from build123d import *

# Parameters (mm, degrees)
F0_W         = 50
F0_H         = 16
F1_DEPTH     = 13
F2_W         = 6.1
F2_H         = 2
F2_H_2       = 16
F3_DEPTH     = 1
F5_D         = 2.5
F5_DEPTH     = 9.5
F5_TIP       = 0.7510757738
F6_SIZE      = 0.5
F8_DEPTH     = 50.001
F9_DEPTH     = 50.001
F10_T1_DEPTH = 22.4650386507
F10_T3_DEPTH = 22.5


# Not quite as in the source:
# - a fillet or chamfer that OpenCascade refuses, or shapes differently, is made with other operations: its cross-section is extruded or revolved along the edge and cut away or added


with BuildPart() as f1:
    # F0 (on Front) → F1 (new body)
    with BuildSketch(Plane.XZ):
        with Locations((25, 8)):
            Rectangle(F0_W, F0_H)
    extrude(amount=F1_DEPTH)

    # F2 (on face) → F3 (cut)
    with BuildSketch(Plane.XZ.offset(13)):
        with Locations((24.95, -1)):
            Rectangle(F2_W, F2_H)
        with Locations((24.95, 8)):
            Rectangle(F2_W, F2_H_2)
    extrude(amount=-F3_DEPTH, mode=Mode.SUBTRACT)

    # F5
    with Locations(Plane.XZ.offset(12)):
        with Locations((24.95, 11), (24.95, 2)):
            Hole(F5_D / 2, depth=F5_DEPTH)
            with Locations((0, 0, -(F5_DEPTH + F5_TIP / 2))):  # 118° drill point
                Cone(0, F5_D / 2, F5_TIP, mode=Mode.SUBTRACT)

    # F6
    f6_edges = [f1.edges().sort_by_distance(p)[0] for p in [
        (0, 0, 8),
        (25, 0, 16),
        (25, 0, 0),
    ]]
    chamfer(f6_edges, length=F6_SIZE)

    # F7 (on face) → F8 (cut, through all)
    with BuildSketch(Plane(origin=(0, 0, 0), x_dir=(0, -1, 0), z_dir=(-1, 0, 0))):
        Polygon((0, 3.5), (0, 2.5), (0.5, 3), align=None)
        Polygon((0, 4.5), (0, 3.5), (0.5, 4), align=None)
        Polygon((0, 5.5), (0, 4.5), (0.5, 5), align=None)
        Polygon((0, 6.5), (0, 5.5), (0.5, 6), align=None)
        Polygon((0, 7.5), (0, 6.5), (0.5, 7), align=None)
        Polygon((0, 8.5), (0, 7.5), (0.5, 8), align=None)
        Polygon((0, 9.5), (0, 8.5), (0.5, 9), align=None)
        Polygon((0, 10.5), (0, 9.5), (0.5, 10), align=None)
        Polygon((0, 11.5), (0, 10.5), (0.5, 11), align=None)
        Polygon((0.5, 12), (0, 12.5), (0, 11.5), align=None)
        Polygon((0.5, 13), (0, 13.5), (0, 12.5), align=None)
        Polygon((0.5, 14), (0, 14.5), (0, 13.5), align=None)
        Polygon((0.5, 15), (0, 15.5), (0, 14.5), align=None)
        Polygon((0.5, 16), (0.5349613493, 16), (0, 16.5), (0, 15.5), (0.5, 15.9673234811), align=None)
        Polygon((0.5, 15.9673234811), (0.5349613493, 16), (0.5, 16), align=None)
        Polygon((0, 1.5), (0, 0.5), (0.5, 1), align=None)
    extrude(amount=-F8_DEPTH, mode=Mode.SUBTRACT)

    # F7 (on face) → F9 (cut, through all)
    with BuildSketch(Plane(origin=(0, 0, 0), x_dir=(0, -1, 0), z_dir=(-1, 0, 0))):
        Polygon((0, 2.5), (0, 1.5), (0.5, 2), align=None)
    extrude(amount=-F9_DEPTH, mode=Mode.SUBTRACT)

    # F10: fillet of radius 2 on 4 edges, made by hand

    # F10_s2 → F10_t1 (cut)
    with BuildSketch(Plane.XZ.offset(-4.4650386507)):
        with BuildLine():
            ThreePointArc((48, 16), (49.4142135624, 15.4142135624), (50, 14))
            Line((50, 14), (50, 16))
            Line((50, 16), (48, 16))
        make_face()
        with BuildLine():
            ThreePointArc((0, 14), (0.5857864376, 15.4142135624), (2, 16))
            Line((2, 16), (0, 16))
            Line((0, 16), (0, 14))
        make_face()
    extrude(amount=F10_T1_DEPTH, mode=Mode.SUBTRACT)

    # F10_s4 → F10_t3 (cut)
    with BuildSketch(Plane.XZ.offset(-4.5)):
        with BuildLine():
            ThreePointArc((48, 0), (49.4142135624, 0.5857864376), (50, 2))
            Line((50, 2), (50, 0))
            Line((50, 0), (48, 0))
        make_face()
        with BuildLine():
            ThreePointArc((0, 2), (0.5857864376, 0.5857864376), (2, 0))
            Line((2, 0), (0, 0))
            Line((0, 0), (0, 2))
        make_face()
    extrude(amount=F10_T3_DEPTH, mode=Mode.SUBTRACT)


solid = f1.part
Read the model definition and answer for the solid it produces. Units are mm, in the model's axes. A direction names the side the tool comes from. Coordinates: 2 decimals unless noted, no trailing zeros. Loops run counter-clockwise (first coordinate to the right, second up) from the corner with the lowest first, then second, coordinate; pieces in that order, holes last.
Q1. This flat-tipped pin is pushed along its axis until it touches: pin 1 Ø3 at (x, z) = (24.95, 2) entering from -Y. Where does it stop, or does it pass through?
Q2. Which of the six approach directions +Z, -Z, +X, -X, +Y, -Y give full straight-line access (tool end or side, diameter ignored) to faces 1 (the face through (26.2, -7.18, 11.05)), 2 (the face through (25, -12, 8)), 3 (the face through (0.57, -6.41, 15.4))?
Q3. Consider probe 1 along Z at (x, y) = (24.95, -7); probe 2 along X at (y, z) = (-9.75, 11); probe 3 along X at (y, z) = (-5.25, 10). Determine where each line is inside the solid, lowest interval first.
Q4. The mould has two halves that part along X. Classify faces 4 (the face through (50, -6, 8)), 5 (the face through (21.9, -12.5, 8.1)), 6 (the face through (0.57, -6.41, 0.6)): +X half, -X half, draft (parallel to the pull), parting line (faces both ways), or undercut.
Q5. The part is cut by section A-A on y = -9. Write down the section's boundary in (x, z), and give its area (3 significant figures).
Results below:
1. pin 1: stops at y = -12
2. face 1: -Y
2. face 2: +Z, -Z, -Y
2. face 3: +Z, -X, +Y, -Y
3. probe 1: z = 0 to 0.75, 3.25 to 9.75, 12.25 to 16
3. probe 2: x = 0 to 23.7, 26.2 to 50
3. probe 3: x = 0 to 24.2, 25.7 to 50
4. face 4: +X half
4. face 5: undercut
4. face 6: -X half
5. outline: (0, 2) arc R2 ccw to (2, 0) - (48, 0) arc R2 ccw to (50, 2) - (50, 14) arc R2 ccw to (48, 16) - (2, 16) arc R2 ccw to (0, 14) - close; hole circle Ø2.5 at (24.95, 2); hole circle Ø2.5 at (24.95, 11)
5. area: 787 mm2
